CAD build for the part. Positions are in the model's coordinates, mm. Face numbers are marked on the shaded views. A direction names the side the tool comes from. Round coordinates to 2 decimals unless told otherwise and drop trailing zeros. Order: outer loops, then holes, each group sorted by start corner. A loop starts at its lowest first (then second) coordinate and runs counter-clockwise, first axis right, second up. Notation, with made-up numbers: M 41.5,-5.5 L 50.5,-5.5 A13 cw 50.5,15.5 Z; hole C -33,62 d6. An arc over 180 degrees is marked long. Put each result on its own line as item: value.
```python
from build123d import *

# Parameters (mm, degrees)
SKETCH1_R           = 6.35
BOSS_EXTRUDE1_DEPTH = 57.15
SKETCH3_R           = 6.35
SKETCH3_R_2         = 3.175
CUT_EXTRUDE1_DEPTH  = 12.7


with BuildPart() as part:
    # Sketch1 → Boss-Extrude1 (new body)
    with BuildSketch(Plane.XY):
        Circle(SKETCH1_R)
    extrude(amount=BOSS_EXTRUDE1_DEPTH)

    # Sketch3 → Cut-Extrude1 (cut)
    with BuildSketch(Plane(origin=(0, 0, 0), x_dir=(-1, 0, 0), z_dir=(0, 0, -1))):
        Circle(SKETCH3_R)
        Circle(SKETCH3_R_2, mode=Mode.SUBTRACT)
    cut_extrude1 = extrude(amount=-CUT_EXTRUDE1_DEPTH, mode=Mode.SUBTRACT)

    # Mirror1: Cut-Extrude1 across plane
    add(cut_extrude1.mirror(Plane.XY.offset(28.575)), mode=Mode.SUBTRACT)


solid = part.part
```
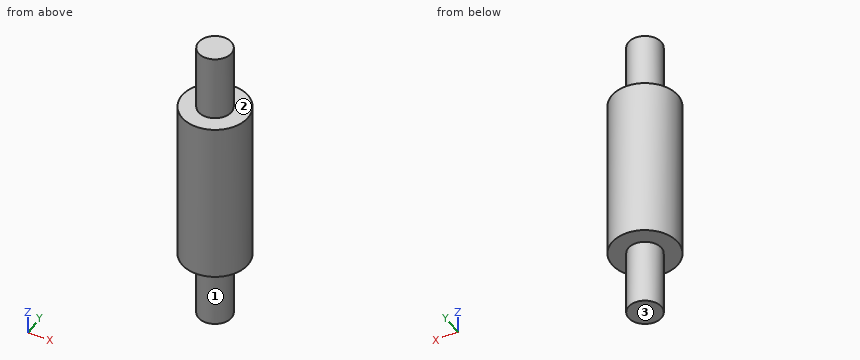
Item 1: Tool access for the marked faces 1, 2 and 3: list every direction of +Z, -Z, +X, -X, +Y, -Y with a clear straight run to the whole face (end or side of a thin tool).
Answers below:
face 1: -Z
face 2: +Z
face 3: -Z, +X, -X, +Y, -Y
Item 2: Pin check, flat tips, straight feed: P1, Ø4, axis at x = -4.5, z = 46, coming from the -Y side; P2, Ø1.5, axis at y = -0.5, z = 39.5, coming from the -X side. Stop position of each tip, or through.
Answers below:
P1: y = -5.46
P2: x = -6.35
Item 3: Band-saw the part on C-C on z = 54. Give the cut face in (x, y) (3 decimals).
Answers below:
outline: C 0,0 d6.35
Item 4: Band-saw the part on D-D on z = 38.5. Give the cut face in (x, y), and give its area (3 significant figures).
Answers below:
outline: C 0,0 d12.7
area: 127 mm²
Item 5: Band-saw the part on A-A on x = 0. Give the cut face in (y, z) (3 decimals), and give its area (3 significant figures).
Answers below:
outline: M -6.35,12.7 L -3.175,12.7 L -3.175,0 L 3.175,0 L 3.175,12.7 L 6.35,12.7 L 6.35,44.45 L 3.175,44.45 L 3.175,57.15 L -3.175,57.15 L -3.175,44.45 L -6.35,44.45 Z
area: 565 mm²
Item 6: Probe line 1 along X through (y, z) = (5.5, 33.5); line 2 along Z through (x, y) = (4, 2); line 3 along X through (y, z) = (-2, 15.5). List the from-to ranges inside material, lowest first. Write a range as [from, to].
Answers below:
line 1: [-3.17, 3.17]
line 2: [12.7, 44.45]
line 3: [-6.03, 6.03]
